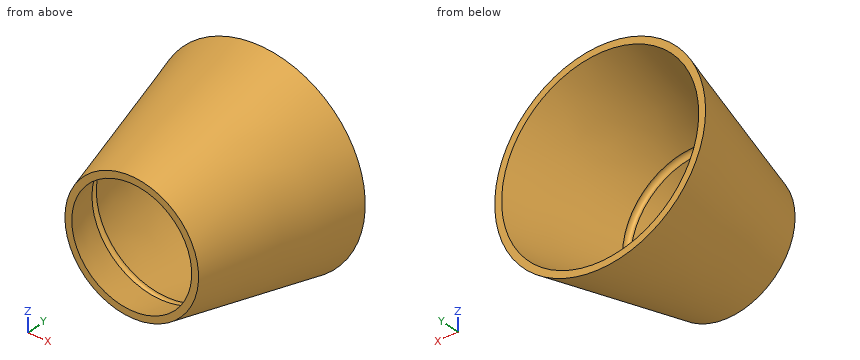
from build123d import *

# Parameters (mm, degrees)
F2_T = -2.5
F3_R = 1.5


with BuildPart() as f1:
    # F0 (on Top) → F1 (revolve)
    with BuildSketch(Plane.XY):
        Polygon((-39.429533, 60), (-25, 0), (0, 0), (0, 60), align=None)
    revolve(axis=Axis((0, 30, 0), (0, -1, 0)))

    # F2
    f2_openings = [f1.faces().sort_by_distance(p)[0] for p in [
        (0, 60, 0),
        (0, 0, 0),
    ]]
    offset(amount=F2_T, openings=f2_openings)

    # F3 (on Right) → F4 (revolve, cut)
    with BuildSketch(Plane.YZ):
        with Locations((15, 26)):
            Circle(F3_R)
    revolve(axis=Axis((0, 19.297946, 0), (0, 1, 0)), mode=Mode.SUBTRACT)


solid = f1.part
CAD build for the part. Positions are in the model's coordinates, mm. Coordinates: 2 decimals unless noted, no trailing zeros. Loops run counter-clockwise (first coordinate to the right, second up) from the corner with the lowest first, then second, coordinate; pieces in that order, holes last. Notation, with made-up numbers: (-19.75, 14.25) - (11.25, 14.25) arc R23 ccw to (11.25, 50.25) - close; hole circle Ø1 at (45.25, 56.25). An arc over 180 degrees is marked (long way). Write item = value, one per line. Start each with the question number.
Q1. Flat gauge pins, fed straight in: pin 1 Ø3 at (y, z) = (42.5, 9.5) entering from +X; pin 2 Ø1 at (y, z) = (21.5, -21) entering from +X; pin 3 Ø1 at (x, y) = (30, 39) entering from -Z. Where does each tip first touch, or does it go through?
Q2. Cut at D-D, the plane y = 9.5. List the corners of the cut face in (x, z).
Q3. Cut at B-B, the plane x = 0. List the corners of the cut face in (y, z).
Q4. Cut at C-C, the plane y = 38. List the corners of the cut face in (x, z), then the cut area to 3 significant figures.
Q5. Drill centre lines: L1, parallel to X at y = 9.5, z = 4; L2, parallel to Z at x = 13.5, y = 37.5; L3, parallel to X at y = 28.5, z = 1. Where is each one in solid material? Low to high.
Q6. Cut at A-A, the plane z = 0. List the corners of the cut face in (x, y).
Computed:
q1.pin_1 = 34.46
q1.pin_2 = 22.16
q1.pin_3 = -17.69
q2.outline = circle Ø54.57 at (0, 0); hole circle Ø49.43 at (0, 0)
q3.outline = (0, -25) - (60, -39.43) - (60, -36.86) - (16.45, -26.38) arc R1.5 cw to (13.53, -25.68) - (0, -22.43) - close; (0, 22.43) - (13.53, 25.68) arc R1.5 cw to (16.45, 26.38) - (60, 36.86) - (60, 39.43) - (0, 25) - close
q4.outline = circle Ø68.28 at (0, 0); hole circle Ø63.13 at (0, 0)
q4.area = 531 mm²
q5.L1 = -26.99 to -24.39, 24.39 to 26.99
q5.L2 = -31.23 to -28.4, 28.4 to 31.23
q5.L3 = -31.84 to -29.27, 29.27 to 31.84
q6.outline = (-39.43, 60) - (-25, 0) - (-22.43, 0) - (-25.68, 13.53) arc R1.5 cw to (-26.38, 16.45) - (-36.86, 60) - close; (22.43, 0) - (25, 0) - (39.43, 60) - (36.86, 60) - (26.38, 16.45) arc R1.5 cw to (25.68, 13.53) - close
